from build123d import *

# Parameters (mm, degrees)
SKETCH1_W                                  = 120
SKETCH1_H                                  = 120
SKETCH1_R                                  = 2.5
BOSS_EXTRUDE1_DEPTH                        = 3
FILLET1_R                                  = 5
SKETCH2_R                                  = 1.5
CUT_EXTRUDE1_DEPTH                         = 85.905830189
MIRROR3_AT_THE_SECOND_PLANE_COPY_1_SKETC_R = 1.5
MIRROR3_AT_THE_SECOND_PLANE_COPY_1_DEPTH   = 85.905830189
SKETCH3_R                                  = 1.7
CUT_EXTRUDE2_DEPTH                         = 85.905830189


with BuildPart() as part:
    # Sketch1 → Boss-Extrude1 (new body)
    with BuildSketch(Plane(origin=(0, 0, 0), x_dir=(1, 0, 0), z_dir=(0, 1, 0))):
        Rectangle(SKETCH1_W, SKETCH1_H)
        with Locations(Location((-7.5, -8, 0), (0, 0, 270))):
            Circle(SKETCH1_R, mode=Mode.SUBTRACT)
        with Locations(Location((7.5, 8, 0), (0, 0, 270))):
            Circle(SKETCH1_R, mode=Mode.SUBTRACT)
        with Locations(Location((7.5, -8, 0), (0, 0, 270))):
            Circle(SKETCH1_R, mode=Mode.SUBTRACT)
        with Locations(Location((-7.5, 8, 0), (0, 0, 270))):
            Circle(SKETCH1_R, mode=Mode.SUBTRACT)
    extrude(amount=BOSS_EXTRUDE1_DEPTH)

    # Fillet1
    fillet1_edges = [part.edges().sort_by_distance(p)[0] for p in [
        (60, 1.5, 60),
        (-60, 1.5, 60),
        (-60, 1.5, -60),
        (60, 1.5, -60),
    ]]
    fillet(fillet1_edges, radius=FILLET1_R)

    # Sketch2 → Cut-Extrude1 (cut, through all)
    with BuildSketch(Plane(origin=(0, 3, 0), x_dir=(1, 0, 0), z_dir=(0, 1, 0))):
        with Locations(Location((-55, 55, 0), (0, 0, 270))):
            Circle(SKETCH2_R)
    cut_extrude1 = extrude(amount=-CUT_EXTRUDE1_DEPTH, mode=Mode.SUBTRACT)

    # Mirror3: Cut-Extrude1 across plane
    add(cut_extrude1.mirror(Plane.XY), mode=Mode.SUBTRACT)

    # Mirror3 at the second plane: Cut-Extrude1 across plane
    add(cut_extrude1.mirror(Plane(origin=(0, 0, 0), x_dir=(0, 0, 1), z_dir=(1, 0, 0))), mode=Mode.SUBTRACT)

    # Mirror3 at the second plane copy 1 sketc → Mirror3 at the second plane copy 1 (cut, through all)
    with BuildSketch(Plane(origin=(0, 3, 0), x_dir=(-1, 0, 0), z_dir=(0, 1, 0))):
        with Locations(Location((-55, 55, 0), (0, 0, 270))):
            Circle(MIRROR3_AT_THE_SECOND_PLANE_COPY_1_SKETC_R)
    extrude(amount=-MIRROR3_AT_THE_SECOND_PLANE_COPY_1_DEPTH, mode=Mode.SUBTRACT)

    # Sketch3 → Cut-Extrude2 (cut, through all)
    with BuildSketch(Plane(origin=(0, 3, 0), x_dir=(1, 0, 0), z_dir=(0, 1, 0))):
        with Locations(Location((20, 21, 0), (0, 0, 270))):
            Circle(SKETCH3_R)
        with Locations(Location((20, -21, 0), (0, 0, 270))):
            Circle(SKETCH3_R)
    extrude(amount=-CUT_EXTRUDE2_DEPTH, mode=Mode.SUBTRACT)


solid = part.part
The model under review builds one solid part; all positions refer to its coordinate system, in mm. Coordinates: 2 decimals unless noted, no trailing zeros. Loops run counter-clockwise (first coordinate to the right, second up) from the corner with the lowest first, then second, coordinate; pieces in that order, holes last. Notation, with made-up numbers: M 24,87 L 79,87 A26 cw 79,107 Z; hole C 26.5,-34.75 d10. An arc over 180 degrees is marked long. Put each result on its own line as item: value. Start each with the question number.
Q1. Add section A-A (z = 21). Write out the cut boundary in (x, y).
Q2. Add section C-C (x = 20). Write out the cut boundary in (y, z).
Q3. Clearance check with a flat-ended pin moving along its axis: pin 1 (2.5 mm diameter, centred on x = -55, z = 55, fed in from -Y). State where the tip first meets the part, or that it passes through.
Q4. The part is to be moulded in two halves that separate along X. For faces 1 (the cylindrical face through (54.55, 1.52, 53.57)), 2 (the cylindrical face through (-54.55, 1.52, -53.57)), 3 (the flat face through (60, 1, 1)), 4 (the flat face through (-1, 1, -60)), say which applies: +X half, -X half, draft (parallel to the pull), parting line (faces both ways), or undercut.
Q5. Wall thickness on line 1 (X direction, y = 1.15, z = -55); line 2 (X direction, y = 1.75, z = 8): over which ranges is each line inside the solid? List them lowest first.
Q6. Add section B-B (x = -7.5). Write out the cut boundary in (y, z), and give its area (3 significant figures).
Answers:
1. outline: M -60,0 L 18.3,0 L 18.3,3 L -60,3 Z; M 21.7,0 L 60,0 L 60,3 L 21.7,3 Z
2. outline: M 0,-60 L 3,-60 L 3,-22.7 L 0,-22.7 Z; M 0,-19.3 L 3,-19.3 L 3,19.3 L 0,19.3 Z; M 0,22.7 L 3,22.7 L 3,60 L 0,60 Z
3. pin 1: passes through
4. face 1: undercut
4. face 2: undercut
4. face 3: +X half
4. face 4: draft
5. line 1: x = -60 to -56.5, -53.5 to 53.5, 56.5 to 60
5. line 2: x = -60 to -10, -5 to 5, 10 to 60
6. outline: M 0,-60 L 3,-60 L 3,-10.5 L 0,-10.5 Z; M 0,-5.5 L 3,-5.5 L 3,5.5 L 0,5.5 Z; M 0,10.5 L 3,10.5 L 3,60 L 0,60 Z
6. area: 330 mm^2
